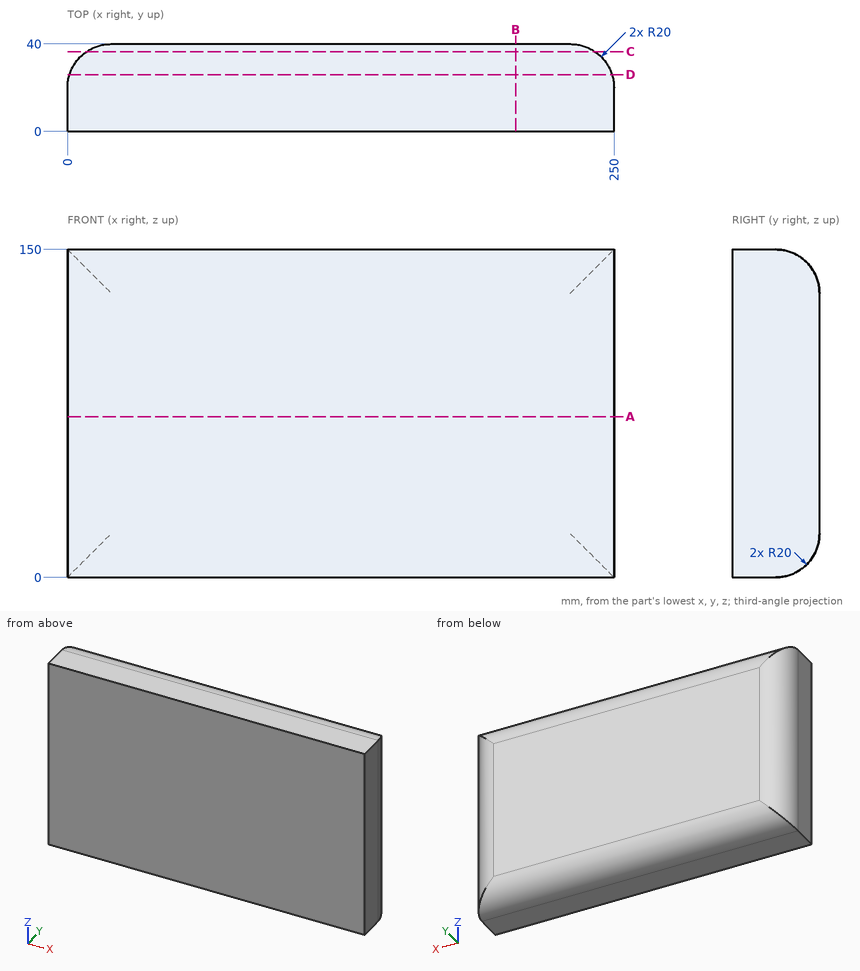
Verification items for this drawing (mm, ordinates from the low corner). Round coordinates to 2 decimals unless told otherwise and drop trailing zeros. Loops run counter-clockwise (first coordinate to the right, second up) from the corner with the lowest first, then second, coordinate; pieces in that order, holes last. Notation, with made-up numbers: (22, 27) -> (26, 27) arc R19 cw to (26, 45) -> close; hole circle Ø7 at (57, 41). An arc over 180 degrees is marked (long way). Answer in a Markdown table with one row per item.
Q1. Thickness scan on L1, parallel to Z at x = 209.5, y = 21; L2, parallel to X at y = 21.5, z = 23; L3, parallel to Z at x = 159, y = 32. Record the ranges inside material, lowest first.
Data:
| item | result |
|---|---|
| L1 | z = 0.03 to 149.97 |
| L2 | x = 0.06 to 249.94 |
| L3 | z = 4 to 146 |
Q2. Sectioned sample at A-A on z = 73.5. Enter the section's corners in (x, y).
Data:
| item | result |
|---|---|
| outline | (0, 0) -> (250, 0) -> (250, 20) arc R20 ccw to (230, 40) -> (20, 40) arc R20 ccw to (0, 20) -> close |
Q3. Go/stop test with flat-tipped pins: P1, Ø1, axis at y = 36, z = 75, coming from the -X side; P2, Ø3, axis at x = 173, z = 86.5, coming from the -Y side; P3, Ø1, axis at x = 206, y = 23, coming from the +Z side; P4, Ø1.5, axis at x = 41.5, y = 30.5, coming from the -Z side. Record where each tip stops, or that it passes through.
Data:
| item | result |
|---|---|
| P1 | stops at x = 7.36 |
| P2 | stops at y = 0 |
| P3 | stops at z = 149.84 |
| P4 | stops at z = 2.54 |
Q4. Sectioned sample at C-C on y = 36.5. Enter the section's corners in (x, z).
Data:
| item | result |
|---|---|
| outline | (8.7, 8.7) -> (241.3, 8.7) -> (241.3, 141.3) -> (8.7, 141.3) -> close |
Q5. Sectioned sample at D-D on y = 26. Enter the section's corners in (x, z), then the cut area to 3 significant figures.
Data:
| item | result |
|---|---|
| outline | (0.92, 0.92) -> (249.08, 0.92) -> (249.08, 149.08) -> (0.92, 149.08) -> close |
| area | 36,800 mm^2 |
Q6. Sectioned sample at B-B on x = 205. Enter the section's corners in (y, z), then the cut area to 3 significant figures.
Data:
| item | result |
|---|---|
| outline | (0, 0) -> (20, 0) arc R20 ccw to (40, 20) -> (40, 130) arc R20 ccw to (20, 150) -> (0, 150) -> close |
| area | 5,830 mm^2 |
